```python
from build123d import *

# Parameters (mm, degrees)
ESBO_O1_W                = 92
ESBO_O1_H                = 62
RESSALTO_EXTRUS_O1_DEPTH = 26
FILETE1_R                = 2
CASCA2_START             = -44
CASCA2_OUTLINE_W         = 22
CASCA2_OUTLINE_H         = 58
CASCA2_DEPTH             = 88


# Read off the part's stored shape, not the designer's step: Casca2
with BuildPart() as part:
    # Esboço1 → Ressalto-extrusão1 (new body)
    with BuildSketch(Plane(origin=(0, 0, 0), x_dir=(1, 0, 0), z_dir=(0, 1, 0))):
        Rectangle(ESBO_O1_W, ESBO_O1_H)
    extrude(amount=RESSALTO_EXTRUS_O1_DEPTH)

    # Filete1
    filete1_edges = [part.edges().sort_by_distance(p)[0] for p in [
        (-46, 26, 0),
        (0, 26, 31),
        (46, 26, 0),
        (0, 0, 31),
        (-46, 0, 0),
        (0, 0, -31),
        (46, 0, 0),
        (0, 26, -31),
        (46, 13, 31),
        (-46, 13, 31),
        (-46, 13, -31),
        (46, 13, -31),
    ]]
    fillet(filete1_edges, radius=FILETE1_R)

    # Casca2 outline → Casca2 (cut)
    with BuildSketch(Plane.YZ.offset(CASCA2_START)):
        with Locations((13, 0)):
            Rectangle(CASCA2_OUTLINE_W, CASCA2_OUTLINE_H)
    extrude(amount=CASCA2_DEPTH, mode=Mode.SUBTRACT)


solid = part.part
```
Can you work these out from the model? Positions are in its coordinate system, mm. A direction names the side the tool comes from. Coordinates: 2 decimals unless noted, no trailing zeros. Loops run counter-clockwise (first coordinate to the right, second up) from the corner with the lowest first, then second, coordinate; pieces in that order, holes last. Notation, with made-up numbers: (49.25, 74.5) -> (102.25, 74.5) arc R30 ccw to (102.25, 106.5) -> close; hole circle Ø9 at (-4, -39.75). An arc over 180 degrees is marked (long way). Put each result on its own line as item: value. Start each with the question number.
Q1. I want a section at A-A (y = 10.25). Write out the boundary of the cut face in (x, z), plus the area to 3 significant figures.
Q2. For faces 4 (the face through (-1, 2, 0)), 5 (the face through (-45.43, 0.6, -0.41)), which set-ups out of +Z, -Z, +X, -X, +Y, -Y let a thin tool reach every point of the face, with its end or its side?
Q3. I want a section at B-B (z = 18). Write out the boundary of the cut face in (x, y), plus the area to 3 significant figures.
Q4. Thinking about a two-plate mould opening in Z: for faces 1 (the face through (45.4, 13.15, 30.43)), 2 (the face through (-1, 13, -31)), 3 (the face through (-1, 13, 29)), which applies, pulls with the +Z half, pulls with the -Z half, needs draft (parallel to the pull), parting line crosses it, or undercut?
Q5. If I drill on line 1 (Z direction, x = 3, y = 8.5); line 2 (X direction, y = 15, z = -8.5); line 3 (Y direction, x = 36, z = -24), over which ranges is the centre line in solid material (lowest first)? Write a range as [from, to].
Taken from the geometry:
1. outline: (-46, -29) arc R2 ccw to (-44, -31) -> (44, -31) arc R2 ccw to (46, -29) -> (46, 29) arc R2 ccw to (44, 31) -> (-44, 31) arc R2 ccw to (-46, 29) -> close; hole (-44, -29) -> (44, -29) -> (44, 29) -> (-44, 29) -> close
1. area: 597 mm2
2. face 4: none
2. face 5: +Z, -Z, -X, -Y
3. outline: (-46, 2) arc R2 ccw to (-44, 0) -> (44, 0) arc R2 ccw to (46, 2) -> (46, 24) arc R2 ccw to (44, 26) -> (-44, 26) arc R2 ccw to (-46, 24) -> close; hole (-44, 2) -> (44, 2) -> (44, 24) -> (-44, 24) -> close
3. area: 453 mm2
4. face 1: pulls with the +Z half
4. face 2: pulls with the -Z half
4. face 3: undercut
5. line 1: z = [-31, -29], [29, 31]
5. line 2: x = [-46, -44], [44, 46]
5. line 3: y = [0, 2], [24, 26]
